from build123d import *

# Parameters (mm, degrees)
F0_W     = 138.43
F0_H     = 139.7
F1_DEPTH = 38.1
F3_DEPTH = 139.701
F4_W     = 133.35
F4_H     = 134.62
F5_DEPTH = 36.7350705877
F6_W     = 134.5792934299
F6_H     = 136.8863768876
F7_DEPTH = 2.54


with BuildPart() as f1:
    # F0 (on Top) → F1 (new body)
    with BuildSketch(Plane.XY):
        with Locations((-10.2020979563, 16.2360354245)):
            Rectangle(F0_W, F0_H)
    extrude(amount=F1_DEPTH)

    # F2 (on face) → F3 (cut, through all)
    with BuildSketch(Plane.XZ.offset(53.6139645755)):
        Polygon((59.0129020437, 38.1), (-79.4170979563, 38.1), (59.0129020437, 0), align=None)
    extrude(amount=-F3_DEPTH, mode=Mode.SUBTRACT)

    # F4 (on face) → F5 (cut, through all)
    with BuildSketch(Plane(origin=(4.1555130146, 0, 15.098363953), x_dir=(0.9641488343, 0, -0.2653620645), z_dir=(0.2653620645, 0, 0.9641488343))):
        with Locations((-13.5877792845, 16.2360354245)):
            Rectangle(F4_W, F4_H)
    extrude(amount=-F5_DEPTH, mode=Mode.SUBTRACT)

    # F6 (on Top) → F7 (join)
    with BuildSketch(Plane.XY):
        with Locations((-10.9574608505, 15.957294032)):
            Rectangle(F6_W, F6_H)
    extrude(amount=F7_DEPTH)


solid = f1.part
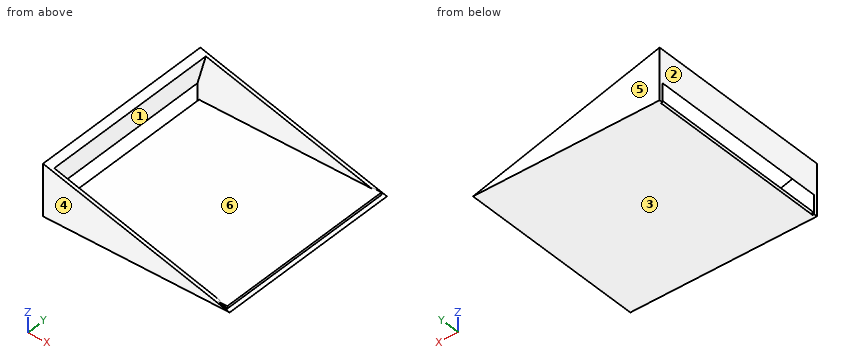
Work out the finished part from the listing and answer in its coordinate system (mm). Face numbers are marked on the shaded views. A direction names the side the tool comes from. Round coordinates to 2 decimals unless told otherwise and drop trailing zeros. Loops run counter-clockwise (first coordinate to the right, second up) from the corner with the lowest first, then second, coordinate; pieces in that order, holes last. Notation, with made-up numbers: (3.25, 32.5) - (28.25, 32.5) arc R19 ccw to (28.25, 52.5) - close; hole circle Ø1 at (66.25, 81). An arc over 180 degrees is marked (long way). One line per item, written item: value.
Q1. Find section A-A on y = 0.5. Give the vertices of the cut face in (x, z).
Check values:
outline: (-79.42, 13.92) - (-73.23, 36.4) - (-79.42, 38.1) - close; (-78.25, 0) - (59.01, 0) - (56.33, 0.74) - (56.33, 2.54) - (-78.25, 2.54) - close
Q2. Find section B-B on z = 5. Give the vertices of the cut face in (x, y).
Check values:
outline: (-79.42, -53.61) - (40.85, -53.61) - (40.85, -51.07) - (-79.42, -51.07) - close; (-79.42, 83.55) - (40.85, 83.55) - (40.85, 86.09) - (-79.42, 86.09) - close
Q3. For the marked faces 1 and 2, determine the directions among +Z, -Z, +X, -X, +Y, -Y from which every point of the face is accessible in a straight line to the end or side of a thin tool.
Check values:
face 1: +X
face 2: +Z, -Z, -X, +Y, -Y
Q4. Find section D-D on z = 23. Give the vertices of the cut face in (x, y), and give its area (3 significant figures).
Check values:
outline: (-79.42, -53.61) - (-24.55, -53.61) - (-24.55, -51.07) - (-76.92, -51.07) - (-76.92, 83.55) - (-24.55, 83.55) - (-24.55, 86.09) - (-79.42, 86.09) - close
area: 615 mm2
Q5. Each of these flat-tipped pins is pushed along its axis until it touches: pin 1 Ø3 at (y, z) = (32.5, 6) entering from +X; pin 2 Ø1.5 at (x, z) = (-4, 18) entering from +Y; pin 3 Ø1.4 at (y, z) = (-0.5, 1.5) entering from +X; pin 4 Ø2 at (y, z) = (-11, 2) entering from -X. Where does it stop, or does it pass through?
Check values:
pin 1: through
pin 2: y = 86.09
pin 3: x = 56.33
pin 4: x = -78.25
Q6. Find section C-C on x = 43. Give the vertices of the cut face in (y, z), and give its area (3 significant figures).
Check values:
outline: (-53.61, 0) - (86.09, 0) - (86.09, 4.41) - (83.55, 4.41) - (83.55, 2.54) - (-51.07, 2.54) - (-51.07, 4.41) - (-53.61, 4.41) - close
area: 364 mm2
Q7. Straight lines are drawn through the part: probe 1 along Y at (x, z) = (-69, 28); probe 2 along Z at (x, y) = (-60, -5.5); probe 3 along X at (y, z) = (61, 20). For each, find the intervals that lie inside material, in ascending order.
Check values:
probe 1: -53.61 to -51.07, 83.55 to 86.09
probe 2: 0 to 2.54
probe 3: -79.42 to -77.74
Q8. The mould has two halves that part along Y. Classify the marked faces 3, 4, 5 and 6: +Y half, -Y half, draft (parallel to the pull), parting line (faces both ways), or undercut.
Check values:
face 3: draft
face 4: -Y half
face 5: +Y half
face 6: undercut
